CAD build for the part. Positions are in the model's coordinates, mm. Face numbers are marked on the shaded views. A direction names the side the tool comes from. Round coordinates to 2 decimals unless told otherwise and drop trailing zeros. Write each loop counter-clockwise with the first axis right and the second up, starting at its lowest first coordinate (ties: lowest second). Pieces come first, ordered by that corner, then holes. Notation, with made-up numbers: (-29, 71.25) -> (-12, 71.25) arc R17 ccw to (-12, 86.25) -> close; hole circle Ø2 at (-8, 51). An arc over 180 degrees is marked (long way). Put each result on its own line as item: value. Start each with the question number.
1. Saw through at A-A on x = 0. List the corners of the cut face in (y, z).
2. Saw through at D-D on x = 3. List the corners of the cut face in (y, z), and give its area (3 significant figures).
3. Drill centre lines: line 1 (Y direction, x = 3.25, z = 2.5); line 2 (X direction, y = 4.7, z = -0.5); line 3 (Y direction, x = 0.25, z = -1.25). Where is each one in solid material? Low to high. Write a range as from..to.
4. 3-axis set-ups, long thin cutter, end or side, ignore diameter. For the marked faces 1 and 2: which of +Z, -Z, +X, -X, +Y, -Y reach the whole face in a straight line?
5. Saw through at C-C on y = 3.5. List the corners of the cut face in (x, z), and give its area (3 significant figures).
6. Saw through at B-B on z = 0.5. List the corners of the cut face in (x, y).
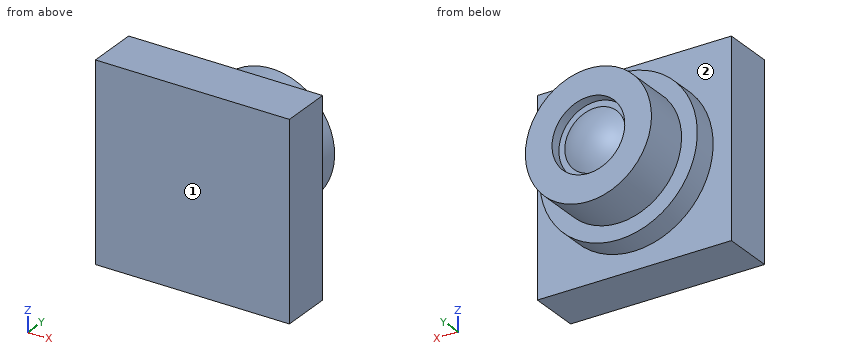
from build123d import *

# Parameters (mm, degrees)
SKETCH1_W           = 8
SKETCH1_H           = 8
BOSS_EXTRUDE1_DEPTH = 2.1


with BuildPart() as part:
    # Sketch1 → Boss-Extrude1 (new body)
    with BuildSketch(Plane(origin=(0, 0, 0), x_dir=(1, 0, 0), z_dir=(0, 1, 0))):
        Rectangle(SKETCH1_W, SKETCH1_H)
    extrude(amount=BOSS_EXTRUDE1_DEPTH)

    # Sketch2 → Revolve1 (revolve)
    with BuildSketch(Plane(origin=(0, 0, 0), x_dir=(0, 0, -1), z_dir=(1, 0, 0)), mode=Mode.PRIVATE) as revolve1_sk:
        with BuildLine():
            Line((-3.25, 2.1), (-3.25, 3.1))
            Line((-3.25, 3.1), (-2.6, 3.1))
            Line((-2.6, 3.1), (-2.6, 5))
            Line((-2.6, 5), (-1.5, 5))
            Line((-1.5, 5), (-1.5, 4.568074784))
            Line((-1.5, 4.568074784), (-1.255377615, 4.568074784))
            ThreePointArc((-1.255377615, 4.568074784), (-0.663801994, 4.888999279), (0, 5))
            Line((0, 5), (0, 2.1))
            Line((0, 2.1), (-3.25, 2.1))
        make_face()
    revolve(revolve1_sk.sketch.rotate(Axis((0, 0, 0), (0, 1, 0)), 180), axis=Axis((0, 0, 0), (0, 1, 0)))


solid = part.part
Return value:
1. outline: (0, -4) -> (2.1, -4) -> (2.1, -3.25) -> (3.1, -3.25) -> (3.1, -2.6) -> (5, -2.6) -> (5, -1.5) -> (4.57, -1.5) -> (4.57, -1.26) arc R2.04 ccw to (4.57, 1.26) -> (4.57, 1.5) -> (5, 1.5) -> (5, 2.6) -> (3.1, 2.6) -> (3.1, 3.25) -> (2.1, 3.25) -> (2.1, 4) -> (0, 4) -> close
2. outline: (0, -4) -> (2.1, -4) -> (2.1, -1.25) -> (3.1, -1.25) -> (3.1, 1.25) -> (2.1, 1.25) -> (2.1, 4) -> (0, 4) -> close
2. area: 19.3 mm^2
3. line 1: y = 0..2.1
3. line 2: x = -2.55..-1.41, -0.94..0.94, 1.41..2.55
3. line 3: y = 0..4.57
4. face 1: +Z, -Z, +X, -X, -Y
4. face 2: +Y
5. outline: circle Ø5.2 at (0, 0)
5. area: 21.2 mm^2
6. outline: (-4, 0) -> (4, 0) -> (4, 2.1) -> (3.21, 2.1) -> (3.21, 3.1) -> (2.55, 3.1) -> (2.55, 5) -> (1.41, 5) -> (1.41, 4.57) -> (1.15, 4.57) arc R1.98 ccw to (-1.15, 4.57) -> (-1.41, 4.57) -> (-1.41, 5) -> (-2.55, 5) -> (-2.55, 3.1) -> (-3.21, 3.1) -> (-3.21, 2.1) -> (-4, 2.1) -> close
